Autodesk Inventor part; units mm, degrees
ref_plane "Work Plane1" through (55, 0, 6) normal (1, 0, 0) x (0, 0, -1)
ref_plane "YZ Plane" through (0, 0, 0) normal (1, 0, 0) x (0, 1, 0)
ref_plane "XZ Plane" through (0, 0, 0) normal (0, 1, 0) x (-1, 0, 0)
sketch "Sketch1" plane through (0, 0, 0) normal (0, 0, 1) x (1, 0, 0)
  line L0 (-32.5, 0) -> (0, 0)
  line L1 (0, 0) -> (0, 54.05)
  line L2 (0, 54.05) -> (110, 54.05)
  line L3 (110, 54.05) -> (110, 0)
  line L4 (110, 0) -> (142.5, 0)
  line L5 (142.5, 0) -> (142.5, -35)
  line L6 (142.5, -35) -> (112.5, -35)
  line L7 (112.5, -35) -> (97.5, -20)
  line L8 (97.5, -20) -> (12.5, -20)
  line L9 (12.5, -20) -> (-2.5, -35)
  line L10 (-2.5, -35) -> (-32.5, -35)
  line L11 (-32.5, -35) -> (-32.5, 0)
  dimension "d0" = 135
  dimension "d1" = 135
  dimension "d2" = 110
  dimension "d3" = 54.05
  dimension "d4" = 35
  dimension "d5" = 32.5
  dimension "d6" = 20
  dimension "d7" = 30
extrude "Extrusion1" add sketch "Sketch1" along normal blind 6
chamfer "Chamfer1" distance 5 angle 45 4 edges at (0, 54.05, 3) (110, 54.05, 3) (-32.5, -35, 3) (142.5, -35, 3)
sketch "Sketch2" plane through (110, 0, 0) normal (0, 1, 0) x (1, 0, 0)
  circle A0 centre (-138.5, 2.5) radius 1.5
  circle A1 centre (-115.5, 2.5) radius 1.5
  line L0 (-142.5, 0) -> (-142.5, -6)
  line L1 (-110, 0) -> (-142.5, 0)
  circle A2 centre (-138.5, 2.5) radius 4
  line L2 (-142.5, 0) -> (-112.5, 0)
  arc A3 (-142.5, 0) -> (-142.3846, 1.5461) centre (-144.8125, 0.95) ccw
  arc A4 (-134.5, 2.5) -> (-132, 0) centre (-132, 2.5) ccw
  arc A5 (-122, 0) -> (-119.5, 2.5) centre (-122, 2.5) ccw
  arc A6 (-111.5, 2.5) -> (-109, 0) centre (-109, 2.5) ccw
  circle A7 centre (-115.5, 2.5) radius 4
  line L3 (-109, 0) -> (-112.3775, 0)
  line L4 (-112.5, 0) -> (-97.5, 0)
  point P0 (-122, 0)
  point P1 (-132, 0)
  point P2 (-118.6225, 0)
  point P3 (-112.3775, 0)
  dimension "d13" = 3
  dimension "d14" = 3
  dimension "d15" = 4
  dimension "d16" = 27
  dimension "d17" = 2.5
  dimension "d18" = 8
extrude "Extrusion2" add sketch "Sketch2" against normal blind 4 contours L1 A2 A4 | L1 A7 A6 L3 | L1 A7 | L1 A5 A7 | L1 A2 | L1 A3 A2 picked at (-115.6011, 0.337) picked at (-138.4397, 0.337)
sketch "Sketch3" plane through (0, 0, 0) normal (0, 0, -1) x (-1, 0, 0)
  line L0 (-105, 54.05) -> (-5, 54.05)
  line L1 (0, 49.05) -> (0, 0)
  line L2 (-110, 0) -> (-110, 49.05)
  point P0 (-84, 48.55)
  point P1 (-26, 48.55)
  dimension "d21" = 5.5
  dimension "d22" = 26
  dimension "d23" = 26
hole "Hole1" at (84, 48.55, 0) at (26, 48.55, 0) direction (0, 0, 1) diameter 4 depth 24
sketch "Sketch4" plane through (12.5, -20, 0) normal (0, -1, 0) x (1, 0, 0)
  line L0 (74, 1.5) -> (72.5, 1.5)
  line L1 (72.5, 1.5) -> (72.5, 4.5)
  line L2 (72.5, 4.5) -> (74, 4.5)
  line L3 (74, 4.5) -> (74, 1.5)
  line L4 (77, 1.5) -> (77, 4.5)
  line L5 (-15, 0) -> (-15, 6)
  line L6 (85, 0) -> (85, 6)
  line L7 (53.5, 1.5) -> (52, 1.5)
  line L8 (52, 1.5) -> (52, 4.5)
  line L9 (52, 4.5) -> (53.5, 4.5)
  line L10 (53.5, 4.5) -> (53.5, 1.5)
  line L11 (56.5, 1.5) -> (56.5, 4.5)
  point P0 (-12.5, 0)
  point P1 (72.5, 3)
  point P2 (-15, 3)
  point P3 (77, 3)
  point P4 (74, 3)
  point P5 (53.5, 3)
  point P6 (56.5, 3)
  dimension "d31" = 1.5
  dimension "d32" = 3
  dimension "d33" = 3
  dimension "d35" = 8
  dimension "d36" = 1.5
  dimension "d37" = 3
  dimension "d38" = 3
  dimension "d39" = 16
revolve "Revolution1" cut sketch "Sketch4" angle 360 about axis through (89.5, -20, 1.5) along (0, 0, 1) contours L0 L1 L2 L3
revolve "Revolution2" cut sketch "Sketch4" angle 360 about axis through (69, -20, 1.5) along (0, 0, 1) contours L7 L8 L9 L10
ref_plane "Work Plane1" through (55, 0, 6) normal (1, 0, 0) x (0, 0, -1)
mirror "Mirror1" about plane through (55, 0, 6) normal (1, 0, 0) of "Extrusion2"
sketch "Sketch5" plane through (0, 0, 6) normal (0, 0, 1) x (1, 0, 0)
  circle A0 centre (101.2237, 19.6209) radius 1.6
  circle A1 centre (70.2706, 22.6087) radius 1.6
  circle A2 centre (21.34, -15.4078) radius 1.6
  circle A3 centre (83.2562, -15.291) radius 1.6
  circle A4 centre (6.3179, 48.8175) radius 1.6
  circle A5 centre (70.2706, 22.6087) radius 4
  circle A6 centre (101.2237, 19.6209) radius 4
  circle A7 centre (83.2562, -15.291) radius 4
  circle A8 centre (21.34, -15.4078) radius 4
  circle A9 centre (6.3179, 48.8175) radius 4
  line L0 (109, 0) -> (109, -4)
  line L1 (12.5, -20) -> (97.5, -20)
  line L2 (110, 0) -> (97.5, -20)
  circle A10 centre (26, 48.55) radius 2
  circle A11 centre (84, 48.55) radius 2
  circle A12 centre (26, 48.55) radius 4
  circle A13 centre (84, 48.55) radius 4
  circle A14 centre (84, 48.55) radius 2
  circle A15 centre (26, 48.55) radius 2
  line L3 (105, 54.05) -> (110, 49.05)
  line L4 (105, 54.05) -> (5, 54.05)
  line L5 (0, 49.05) -> (5, 54.05)
  line L6 (0, 49.05) -> (0, 0)
  line L7 (0, 0) -> (-32.5, 0)
  line L8 (-32.5, 0) -> (-32.5, -30)
  line L9 (-27.5, -35) -> (-2.5, -35)
  line L10 (-2.5, -35) -> (12.5, -20)
  line L11 (12.5, -20) -> (97.5, -20)
  line L12 (97.5, -20) -> (112.5, -35)
  line L13 (112.5, -35) -> (137.5, -35)
  line L14 (142.5, -30) -> (142.5, 0)
  line L15 (142.5, 0) -> (110, 0)
  line L16 (110, 0) -> (110, 49.05)
  line L17 (0, 49.05) -> (5, 54.05)
  line L18 (105, 54.05) -> (5, 54.05)
  line L19 (105, 54.05) -> (110, 49.05)
  line L20 (142.5, -30) -> (137.5, -35)
  line L21 (-27.5, -35) -> (-32.5, -30)
  circle A16 centre (6.3179, 48.8175) radius 1.6
  circle A17 centre (21.34, -15.4078) radius 1.6
  circle A18 centre (70.2706, 22.6087) radius 1.6
  circle A19 centre (101.2237, 19.6209) radius 1.6
  circle A20 centre (83.2562, -15.291) radius 1.6
  line L22 (110, 0) -> (110, 49.05)
  line L23 (0, 49.05) -> (0, 0)
  dimension "d41" = 8
  dimension "d82" = 5.5
  dimension "d83" = 5.5
  dimension "d84" = 26
  dimension "d85" = 26
hole "Hole2" at (6.3179, 48.8175, 6) at (70.2706, 22.6087, 6) at (101.2237, 19.6209, 6) at (83.2562, -15.291, 6) at (21.34, -15.4078, 6) direction (0, 0, -1) diameter 4 depth 24
sketch "Sketch6" plane through (0, 0, 0) normal (0, 0, -1) x (-1, 0, 0)
  line L0 (-110, 0) -> (-110, 49.05)
  line L1 (-110, 46.05) -> (-107, 46.05)
  line L2 (-107, 46.05) -> (-91, 46.05)
  line L3 (-91, 46.05) -> (-91, 10)
  line L4 (-91, 10) -> (-95, 10)
  line L5 (-95, 10) -> (-95, 42.05)
  line L6 (-95, 42.05) -> (-110, 42.05)
  line L7 (-110, 0) -> (-110, 49.05)
  line L8 (-12.5, -20) -> (-97.5, -20)
  line L9 (-107, 46.05) -> (-107, 42.05)
  point P0 (0, 0)
  dimension "d49" = 30
  dimension "d50" = 4
  dimension "d51" = 4
  dimension "d55" = 15
  dimension "d68" = 3
  dimension "d69" = 3
extrude "Extrusion3" cut sketch "Sketch6" against normal blind 2
extrude "Extrusion4" cut sketch "Sketch6" against normal through all contours L0 L1 L9 L6
fillet "Fillet1" radius 4 1 edges at (95, 42.05, 1)
fillet "Fillet2" radius 8 1 edges at (91, 46.05, 1)
chamfer "Chamfer2" distance 2 angle 45 2 edges at (93, 10, 0) (107, 44.05, 2)
sketch "Sketch7" plane through (0, 0, 0) normal (0, 0, -1) x (-1, 0, 0)
  circle A0 centre (-125, -26) radius 4
  circle A1 centre (-125, -26) radius 5 construction
  circle A2 centre (-125, -26) radius 9 construction
  line L0 (-112.5, -35) -> (-137.5, -35)
  circle A3 centre (-125, -26) radius 7.5
  point P0 (0, 0)
  point P1 (-125, -35)
  dimension "d70" = 8
  dimension "d71" = 10
  dimension "d72" = 18
  dimension "d75" = 15
extrude "Extrusion5" cut sketch "Sketch7" against normal through all contours A0
extrude "Extrusion6" cut sketch "Sketch7" against normal blind 3 contours A0 | A3
equation "\"d51\" = d50"
equation "\"d61\" = d60 + d50"
equation "\"MotorHeight\" = MotorHeightBase"
properties part number "Motor Side Foot"
Design review of the part built by this model. Coordinates are the model's own, in mm. A direction names the side the tool comes from. Round coordinates to 2 decimals unless told otherwise and drop trailing zeros. Write each loop counter-clockwise with the first axis right and the second up, starting at its lowest first coordinate (ties: lowest second). Pieces come first, ordered by that corner, then holes. Notation, with made-up numbers: (-8.5, 40) -> (3.5, 40) arc R19 ccw to (3.5, 71) -> close; hole circle Ø11 at (3, -20). An arc over 180 degrees is marked (long way). Answer in a Markdown table with one row per item.
Q1. Take a section at D-D, the plane x = 50. State the section outline as (y, z) points, then the cut area to 3 significant figures.
The answers:
| item | result |
|---|---|
| outline | (-20, 0) -> (54.05, 0) -> (54.05, 6) -> (-20, 6) -> close |
| area | 444 mm² |
Q2. Take a section at C-C, the plane x = 125. State the section outline as (y, z) points.
The answers:
| item | result |
|---|---|
| outline | (-35, 0) -> (-33.5, 0) -> (-33.5, 3) -> (-30, 3) -> (-30, 6) -> (-35, 6) -> close; (-22, 3) -> (-18.5, 3) -> (-18.5, 0) -> (0, 0) -> (0, 6) -> (-22, 6) -> close |
Q3. Take a section at A-A, the plane x = 26. State the section outline as (y, z) points.
The answers:
| item | result |
|---|---|
| outline | (-20, 0) -> (46.55, 0) -> (46.55, 6) -> (-20, 6) -> close; (50.55, 0) -> (54.05, 0) -> (54.05, 6) -> (50.55, 6) -> close |
Q4. Draft analysis for pull direction X (two halves, no side actions). For faces 1 (the face through (137, -4, -4)), 2 (the face through (-5.4, -2, -6.5)), 3 (the face through (6.23, 50.816, 2.958)), 4 (the face through (140, -32.5, 3)), state which applies: +X half, -X half, draft (parallel to the pull), parting line (faces both ways), or undercut.
The answers:
| item | result |
|---|---|
| face 1 | draft |
| face 2 | undercut |
| face 3 | undercut |
| face 4 | +X half |
Q5. To check wall thickness, follow L1, parallel to Y at x = 26, z = 1.4; L2, parallel to Z at x = 115.5, y = -3.05; L3, parallel to Z at x = 115, y = -5.5. State the ranges of each line that lie inside material, in increasing order. Write a range as [from, to].
The answers:
| item | result |
|---|---|
| L1 | [-20, 46.55], [50.55, 54.05] |
| L2 | [-6.5, -4], [-1, 6] |
| L3 | [0, 6] |
Q6. For faces 5 (the face through (85.21, -14.86, 2.96)), 6 (the face through (96.203, 40.909, 1.014)), 7 (the face through (110, 21, 3)), 8 (the face through (89.6, -15.5, 3)), list the 3-axis set-ups (+Z, -Z, +X, -X, +Y, -Y) from which the entire face can be reached by the end or side of a thin tool; tool diameter is ignored.
The answers:
| item | result |
|---|---|
| face 5 | +Z, -Z |
| face 6 | -Z |
| face 7 | +Z, -Z, +X, +Y |
| face 8 | none |
Q7. Clearance check with flat-ended pins moving along their axes: pin 1 Ø1.8 at (x, z) = (104, 3.5) entering from -Y; pin 2 Ø0.6 at (y, z) = (16.5, 0.5) entering from +X; pin 3 Ø4 at (x, z) = (-13.5, 1) entering from +Y. State where each tip first meets the part, or that it passes through.
The answers:
| item | result |
|---|---|
| pin 1 | y = -27.4 |
| pin 2 | x = 110 |
| pin 3 | y = 0 |
Q8. Take a section at B-B, the plane y = 2. State the section outline as (x, z) points, then the cut area to 3 significant figures.
The answers:
| item | result |
|---|---|
| outline | (0, 0) -> (110, 0) -> (110, 6) -> (0, 6) -> close |
| area | 660 mm² |
